Can you work these out from the model? Positions are in its coordinate system, mm. A direction names the side the tool comes from. Give positions to 0.01 mm unless a question says otherwise; leave off trailing zeros. Write each loop counter-clockwise with the first axis right and the second up, starting at its lowest first coordinate (ties: lowest second). Pieces come first, ordered by that corner, then holes.
```python
from build123d import *

# Parameters (mm, degrees)
SKETCH_1_W           = 25
SKETCH_1_H           = 37.5
EXTRUDE_1_DEPTH      = 20
FILLET_1_R           = 5
SKETCH_2_W           = 15
SKETCH_2_H           = 7.5
EXTRUDE_2_DEPTH      = 5
EXTRUDE_START        = -20
SKETCH_2_2_W         = 15
SKETCH_2_2_H         = 7.5
EXTRUDE_3_DEPTH      = 5
SKETCH_3_R           = 1.45
CUT_EXTRUDE_1_DEPTH  = 20
SKETCH_4_R           = 3.025
CUT_EXTRUDE_3_DEPTH  = 2.5
CUT_EXTRUDE_START    = -17.5
SKETCH_4_2_R         = 3.025
CUT_EXTRUDE_4_DEPTH  = 2.5
SKETCH_5_W           = 33
SKETCH_5_H           = 13
CUT_EXTRUDE_5_DEPTH  = 5.5
SKETCH_6_W           = 23
SKETCH_6_H           = 13
CUT_EXTRUDE_6_DEPTH  = 18.5
SKETCH_7_R           = 1.45
CUT_EXTRUDE_7_DEPTH  = 14.5
SKETCH_8_W           = 7
SKETCH_8_H           = 2.5
CUT_EXTRUDE_8_DEPTH  = 42.5
SKETCH_9_W           = 12
SKETCH_9_H           = 15
CUT_EXTRUDE_9_DEPTH  = 5
SKETCH_10_W          = 7
SKETCH_10_H          = 32.5
CUT_EXTRUDE_10_DEPTH = 1
CUT_EXTRUDE_START_2  = 15
SKETCH_10_2_W        = 7
SKETCH_10_2_H        = 32.5
CUT_EXTRUDE_11_DEPTH = 1
CUT_EXTRUDE_12_REACH = 40.332
SKETCH_11_R          = 3
SKETCH_12_R          = 4
EXTRUDE_4_DEPTH      = 6
SKETCH_13_W          = 15.131342966
SKETCH_13_H          = 46.669139603
CUT_EXTRUDE_13_DEPTH = 23


with BuildPart() as part:
    # Эскиз1 → Бобышка-Вытянуть1 (new body)
    with BuildSketch(Plane(origin=(0, 0, 0), x_dir=(1, 0, 0), z_dir=(0, 1, 0))):
        Rectangle(SKETCH_1_W, SKETCH_1_H)
    extrude(amount=EXTRUDE_1_DEPTH)

    # Скругление1
    fillet_1_edges = [part.edges().sort_by_distance(p)[0] for p in [
        (-12.5, 20, 0),
        (0, 20, 18.75),
        (12.5, 20, 0),
        (0, 0, 18.75),
        (-12.5, 0, 0),
        (12.5, 0, 0),
        (12.5, 10, 18.75),
        (-12.5, 10, 18.75),
    ]]
    fillet(fillet_1_edges, radius=FILLET_1_R)

    # Эскиз2 → Бобышка-Вытянуть2 (add)
    with BuildSketch(Plane(origin=(0, 20, 0), x_dir=(1, 0, 0), z_dir=(0, 1, 0))):
        with Locations((0, 22.5)):
            Rectangle(SKETCH_2_W, SKETCH_2_H)
    extrude(amount=-EXTRUDE_2_DEPTH)

    # Эскиз2<2> → Бобышка-Вытянуть3 (add)
    with BuildSketch(Plane(origin=(0, 20, 0), x_dir=(1, 0, 0), z_dir=(0, 1, 0)).offset(EXTRUDE_START)):
        with Locations((0, 22.5)):
            Rectangle(SKETCH_2_2_W, SKETCH_2_2_H)
    extrude(amount=EXTRUDE_3_DEPTH)

    # Эскиз3 → Вырез-Вытянуть1 (cut)
    with BuildSketch(Plane(origin=(0, 20, 0), x_dir=(1, 0, 0), z_dir=(0, 1, 0))):
        with Locations(Location((-4.5, 22.5, 0), (0, 0, 270))):
            Circle(SKETCH_3_R)
        with Locations(Location((4.5, 22.5, 0), (0, 0, 270))):
            Circle(SKETCH_3_R)
    extrude(amount=-CUT_EXTRUDE_1_DEPTH, mode=Mode.SUBTRACT)

    # Эскиз4 → Вырез-Вытянуть3 (cut)
    with BuildSketch(Plane(origin=(0, 20, 0), x_dir=(1, 0, 0), z_dir=(0, 1, 0))):
        with Locations((-4.5, 22.5)):
            Circle(SKETCH_4_R)
        with Locations((4.5, 22.5)):
            Circle(SKETCH_4_R)
    extrude(amount=-CUT_EXTRUDE_3_DEPTH, mode=Mode.SUBTRACT)

    # Эскиз4<2> → Вырез-Вытянуть4 (cut)
    with BuildSketch(Plane(origin=(0, 20, 0), x_dir=(1, 0, 0), z_dir=(0, 1, 0)).offset(CUT_EXTRUDE_START)):
        with Locations((-4.5, 22.5)):
            Circle(SKETCH_4_2_R)
        with Locations((4.5, 22.5)):
            Circle(SKETCH_4_2_R)
    extrude(amount=-CUT_EXTRUDE_4_DEPTH, mode=Mode.SUBTRACT)

    # Эскиз5 → Вырез-Вытянуть5 (cut)
    with BuildSketch(Plane.ZY.offset(12.5)):
        with Locations((-0.25, 10)):
            Rectangle(SKETCH_5_W, SKETCH_5_H)
    extrude(amount=-CUT_EXTRUDE_5_DEPTH, mode=Mode.SUBTRACT)

    # Эскиз6 → Вырез-Вытянуть6 (cut)
    with BuildSketch(Plane.ZY.offset(7)):
        with Locations((-0.25, 10)):
            Rectangle(SKETCH_6_W, SKETCH_6_H)
    extrude(amount=-CUT_EXTRUDE_6_DEPTH, mode=Mode.SUBTRACT)

    # Эскиз7 → Вырез-Вытянуть7 (cut)
    with BuildSketch(Plane.ZY.offset(7)):
        with Locations((-13.95, 10)):
            Circle(SKETCH_7_R)
        with Locations((13.45, 10)):
            Circle(SKETCH_7_R)
    extrude(amount=-CUT_EXTRUDE_7_DEPTH, mode=Mode.SUBTRACT)

    # Эскиз8 → Вырез-Вытянуть8 (cut)
    with BuildSketch(Plane(origin=(0, 0, -26.25), x_dir=(-1, 0, 0), z_dir=(0, 0, -1))):
        with Locations((0, 16.25)):
            Rectangle(SKETCH_8_W, SKETCH_8_H)
        with Locations((0, 3.75)):
            Rectangle(SKETCH_8_W, SKETCH_8_H)
    extrude(amount=-CUT_EXTRUDE_8_DEPTH, mode=Mode.SUBTRACT)

    # Эскиз9 → Вырез-Вытянуть9 (cut)
    with BuildSketch(Plane(origin=(0, 0, 11.25), x_dir=(-1, 0, 0), z_dir=(0, 0, -1))):
        with Locations((-2.5, 10)):
            Rectangle(SKETCH_9_W, SKETCH_9_H)
    extrude(amount=-CUT_EXTRUDE_9_DEPTH, mode=Mode.SUBTRACT)

    # Эскиз10 → Вырез-Вытянуть10 (cut)
    with BuildSketch(Plane.XZ.offset(-17.5)):
        Rectangle(SKETCH_10_W, SKETCH_10_H)
    extrude(amount=-CUT_EXTRUDE_10_DEPTH, mode=Mode.SUBTRACT)

    # Эскиз10<2> → Вырез-Вытянуть11 (cut)
    with BuildSketch(Plane.XZ.offset(-17.5).offset(CUT_EXTRUDE_START_2)):
        Rectangle(SKETCH_10_2_W, SKETCH_10_2_H)
    extrude(amount=CUT_EXTRUDE_11_DEPTH, mode=Mode.SUBTRACT)

    # Вырез-Вытянуть12: up to this face of the body (flat: up to its plane)
    cut_extrude_12_end = Plane(part.part.faces().sort_by_distance((-12.5, 10, -17.75))[0])
    # Эскиз11 → Вырез-Вытянуть12 (cut, up to the picked face)
    with BuildSketch(Plane.ZY.offset(7), mode=Mode.PRIVATE) as cut_extrude_12_sk1:
        with Locations((-13.95, 10)):
            Circle(SKETCH_11_R)
    cut_extrude_12_tool1 = split(extrude(cut_extrude_12_sk1.sketch, amount=CUT_EXTRUDE_12_REACH, mode=Mode.PRIVATE), bisect_by=cut_extrude_12_end, keep=Keep.BOTH, mode=Mode.PRIVATE)
    # Эскиз11 → Вырез-Вытянуть12 (cut, up to the picked face)
    with BuildSketch(Plane.ZY.offset(7), mode=Mode.PRIVATE) as cut_extrude_12_sk2:
        with Locations((13.45, 10)):
            Circle(SKETCH_11_R)
    cut_extrude_12_tool2 = split(extrude(cut_extrude_12_sk2.sketch, amount=CUT_EXTRUDE_12_REACH, mode=Mode.PRIVATE), bisect_by=cut_extrude_12_end, keep=Keep.BOTH, mode=Mode.PRIVATE)
    add(cut_extrude_12_tool1.solids().sort_by(Axis((-7, 10, -13.95), (-1, 0, 0)))[0], mode=Mode.SUBTRACT)
    add(cut_extrude_12_tool2.solids().sort_by(Axis((-7, 10, 13.45), (-1, 0, 0)))[0], mode=Mode.SUBTRACT)

    # Эскиз12 → Бобышка-Вытянуть4 (add)
    with BuildSketch(Plane(origin=(12.5, 0, 0), x_dir=(0, 0, -1), z_dir=(1, 0, 0))):
        with Locations(Location((-4.87, 10, 0), (0, 0, 180))):
            Circle(SKETCH_12_R)
    extrude(amount=EXTRUDE_4_DEPTH)

    # Эскиз13 → Вырез-Вытянуть13 (cut)
    with BuildSketch(Plane(origin=(0, 20, 0), x_dir=(1, 0, 0), z_dir=(0, 1, 0))):
        with Locations((-7.565671483, 2.915430198)):
            Rectangle(SKETCH_13_W, SKETCH_13_H)
    extrude(amount=-CUT_EXTRUDE_13_DEPTH, mode=Mode.SUBTRACT)


solid = part.part
```
1) For faces 5 (the face through (7.5, 3, -22)), 6 (the face through (4, 10, 16.25)), 7 (the face through (2, 15, -15)), which set-ups out of +Z, -Z, +X, -X, +Y, -Y let a thin tool reach every point of the face, with its end or its side?
Values follow:
face 5: -Z, +X, +Y, -Y
face 6: -X
face 7: -Z, -X
2) Suppose I cut it at A-A on z = 9.5. Write out the boundary of the cut face in (x, y).
Values follow:
outline: (0, 0) - (7.5, 0) arc R5 ccw to (12.5, 5) - (12.5, 15) arc R5 ccw to (7.5, 20) - (0, 20) - (0, 18.5) - (3.5, 18.5) - (3.5, 16.5) - (11.5, 16.5) - (11.5, 3.5) - (3.5, 3.5) - (3.5, 1.5) - (0, 1.5) - close
3) Suppose I cut it at B-B on x = 4.5. State how many separate pieces and enclosed holes the cut face has, plus the area to 3 significant figures.
Values follow:
separate pieces: 3
enclosed holes: 2
area: 389 mm2
4) For pin 1 Ø0.8 at (y, z) = (16, -24.5) entering from -X; pin 2 Ø1.5 at (x, y) = (16, 9) entering from +Z; pin 3 Ø1.5 at (y, z) = (4, 3) entering from +X, each with a flat end and sliding along its axis, tell me the tip position at first contact or that it passes through.
Values follow:
pin 1: stops at x = 3.5
pin 2: stops at z = 8.86
pin 3: stops at x = 12.49
5) Suppose I cut it at C-C on y = 10. Write out the boundary of the cut face in (x, z), plus the area to 3 significant figures.
Values follow:
outline: (0, -18.75) - (12.5, -18.75) - (12.5, 0.87) - (18.5, 0.87) - (18.5, 8.87) - (12.5, 8.87) - (12.5, 13.75) arc R5 ccw to (7.5, 18.75) - (0, 18.75) - (0, 16.25) - (8.5, 16.25) - (8.5, 11.25) - (11.5, 11.25) - (11.5, -11.75) - (0, -11.75) - (0, -12.5) - (7.5, -12.5) - (7.5, -15.4) - (0, -15.4) - close
area: 183 mm2
6) Please list where these lines run through material, in increasing order: L1, parallel to Y at x = 2, z = -13.95; L2, parallel to Z at x = 4.5, y = 15.7; L3, parallel to Z at x = 4.5, y = 16.
Values follow:
L1: y = 0 to 1.5, 5 to 8.55, 11.45 to 15, 18.5 to 20
L2: z = -26.25 to -23.95, -21.05 to -11.75, 16.25 to 18.7
L3: z = -26.25 to -23.95, -21.05 to -11.75, 16.25 to 18.65
7) Suppose I cut it at D-D on z = -13.95. Write out the boundary of the cut face in (x, y).
Values follow:
outline: (0, 0) - (7.5, 0) arc R5 ccw to (12.5, 5) - (12.5, 15) arc R5 ccw to (7.5, 20) - (0, 20) - (0, 18.5) - (3.5, 18.5) - (3.5, 15) - (0, 15) - (0, 11.45) - (7.5, 11.45) - (7.5, 8.55) - (0, 8.55) - (0, 5) - (3.5, 5) - (3.5, 1.5) - (0, 1.5) - close
8) If we mould it in two halves opening along Y, with no side actions, what happens to faces 1 (the face through (4, 0, -7)), 2 (the face through (11.07, 18.5, -2.73)), 3 (the face through (3.5, 16, -25)), 4 (the face through (4, 10, 18.75))? For each: +Y half, -Y half, draft (parallel to the pull), parting line (faces both ways), or undercut.
Values follow:
face 1: -Y half
face 2: +Y half
face 3: undercut
face 4: draft
